Read the model definition and answer for the solid it produces. Units are mm, in the model's axes. Face numbers are marked on the shaded views. A direction names the side the tool comes from. Give positions to 0.01 mm unless a question says otherwise; leave off trailing zeros. Write each loop counter-clockwise with the first axis right and the second up, starting at its lowest first coordinate (ties: lowest second). Pieces come first, ordered by that corner, then holes. Notation, with made-up numbers: M 76.5,-21.5 L 96.5,-21.5 A18 ccw 96.5,-9.5 Z; hole C 42,35 d7. An arc over 180 degrees is marked long. Answer as CSV lines item,"result". Start each with the question number.
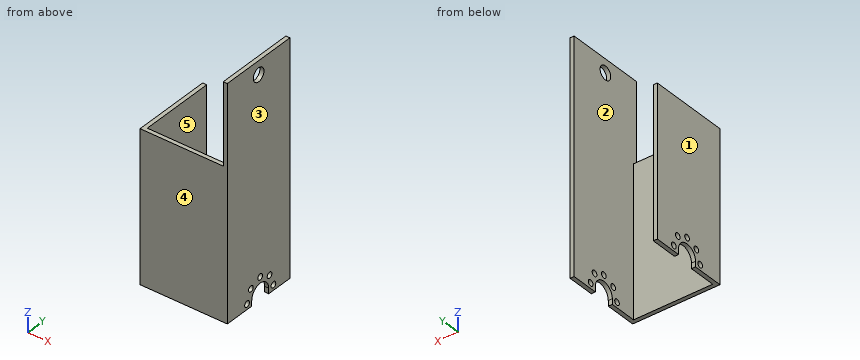
```python
from build123d import *

# Parameters (mm, degrees)
F1_DEPTH  = 28
F2_R      = 1.1
F3_DEPTH  = 32.301
F4_R      = 1.1
F5_DEPTH  = 1.5
F6_W      = 1.5
F6_H      = 86.945
F7_DEPTH  = 32.3
F8_W      = 29.3
F8_H      = 30
F8_W_2    = 1.5
F9_DEPTH  = 29.501
F10_R     = 2.5
F11_DEPTH = 1.5


with BuildPart() as f1:
    # F0 (on Front) → F1 (new body)
    with BuildSketch(Plane.XZ):
        Polygon((0, 86.945), (0, 0), (1.5, 0), (1.5, 85.445), (30.8, 85.445), (30.8, 0), (32.3, 0), (32.3, 86.945), align=None)
    extrude(amount=F1_DEPTH)

    # F2 (on face) → F3 (cut, through all)
    with BuildSketch(Plane(origin=(0, 0, 0), x_dir=(0, -1, 0), z_dir=(-1, 0, 0))):
        with BuildLine():
            Line((18, 0), (18, 2))
            ThreePointArc((18, 2), (14, 6), (10, 2))
            Line((10, 2), (10, 0))
            Line((10, 0), (18, 0))
        make_face()
        with Locations((20.22254, 2)):
            Circle(F2_R)
        with Locations((18.4, 6.4)):
            Circle(F2_R)
        with Locations((14, 8.22254)):
            Circle(F2_R)
        with Locations((9.6, 6.4)):
            Circle(F2_R)
        with Locations((7.77746, 2)):
            Circle(F2_R)
    extrude(amount=-F3_DEPTH, mode=Mode.SUBTRACT)

    # F4 (on face) → F5 (cut, through all)
    with BuildSketch(Plane.XY.offset(86.945)):
        with Locations((6.15, -4)):
            Circle(F4_R)
        with Locations((26.15, -4)):
            Circle(F4_R)
        with Locations((6.15, -24)):
            Circle(F4_R)
        with Locations((26.15, -24)):
            Circle(F4_R)
    extrude(amount=-F5_DEPTH, mode=Mode.SUBTRACT)

    # F6 (on face) → F7 (join)
    with BuildSketch(Plane.YZ.offset(32.3)):
        with Locations((-28.75, 43.4725)):
            Rectangle(F6_W, F6_H)
    extrude(amount=-F7_DEPTH)

    # F8 (on face) → F9 (cut, through all)
    with BuildSketch(Plane.XZ.offset(29.5)):
        with Locations((16.15, 70.445)):
            Rectangle(F8_W, F8_H)
        with Locations((0.75, 70.445)):
            Rectangle(F8_W_2, F8_H)
        Polygon((32.3, 86.945), (0, 86.945), (0, 85.445), (1.5, 85.445), (30.8, 85.445), (32.3, 85.445), align=None)
    extrude(amount=-F9_DEPTH, mode=Mode.SUBTRACT)

    # F10 (on face) → F11 (cut, through all)
    with BuildSketch(Plane.YZ.offset(32.3)):
        with Locations((-14.75, 80.445)):
            Circle(F10_R)
    extrude(amount=-F11_DEPTH, mode=Mode.SUBTRACT)


solid = f1.part
```
1. For the marked faces 4 and 5, determine the directions among +Z, -Z, +X, -X, +Y, -Y from which every point of the face is accessible in a straight line to the end or side of a thin tool.
2. Find the intervals of material crossed by line 1 (Z direction, x = 0.65, y = -9.6) (3 decimals); line 2 (Z direction, x = 31.7, y = -14) (3 decimals); line 3 (X direction, y = -24.5, z = 17), in increasing order. Write a range as [from, to].
3. Given pin 1 (4 mm diameter, centred on x = 15.5, z = 20.5, fed in from +Y), flat-ended and moving along its own axis, determine where the tip first touches the part or whether it passes through.
4. Find section A-A on y = -13.75. Determine the outline of the cut face in (x, z) (3 decimals), then the cut area to 3 significant figures.
5. Find section C-C on x = 24. Determine the outline of the cut face in (y, z) (3 decimals), then the cut area to 3 significant figures.
6. Find section B-B on z = 51. Determine the outline of the cut face in (x, y).
7. Determine the mould class of the marked faces 1, 2 and 3 for opening direction X: +X half, -X half, draft (parallel to the pull), parting line (faces both ways), or undercut.
8. Find section D-D on z = 62.5. Determine the outline of the cut face in (x, y).
Computed:
1,face 4,"+Z, -Z, +X, -X, -Y"
1,face 5,"+Z, -Z, +Y"
2,line 1,"z = [0, 5.3], [7.5, 55.445]"
2,line 2,"z = [6, 7.123], [9.323, 78.06], [82.83, 85.445]"
2,line 3,"x = [0, 1.5], [30.8, 32.3]"
3,pin 1,"stops at y = -28"
4,outline,"M 0,5.992 L 1.5,5.992 L 1.5,7.151 L 0,7.151 Z; M 0,9.294 L 1.5,9.294 L 1.5,55.445 L 0,55.445 Z; M 30.8,5.992 L 32.3,5.992 L 32.3,7.151 L 30.8,7.151 Z; M 30.8,9.294 L 32.3,9.294 L 32.3,78.154 L 30.8,78.154 Z; M 30.8,82.736 L 32.3,82.736 L 32.3,85.445 L 30.8,85.445 Z"
4,area,"180 mm^2"
5,outline,"M -29.5,0 L -28,0 L -28,55.445 L -29.5,55.445 Z"
5,area,"83.2 mm^2"
6,outline,"M 0,-29.5 L 32.3,-29.5 L 32.3,0 L 30.8,0 L 30.8,-28 L 1.5,-28 L 1.5,0 L 0,0 Z"
7,face 1,"-X half"
7,face 2,"undercut"
7,face 3,"+X half"
8,outline,"M 30.8,-29.5 L 32.3,-29.5 L 32.3,0 L 30.8,0 Z"
